Drawing for the job (mm, zero at the part's lowest x, y, z). A direction names the side the tool comes from. Round coordinates to 2 decimals unless told otherwise and drop trailing zeros. Loops run counter-clockwise (first coordinate to the right, second up) from the corner with the lowest first, then second, coordinate; pieces in that order, holes last. Notation, with made-up numbers: M 78,27 L 113,27 A19 cw 113,63 Z; hole C 83.5,7 d3. An arc over 180 degrees is marked long. Use a Markdown table: item, result. Add a question column.
Q1. Pin check, flat tips, straight feed: pin 1 (4 mm diameter, centred on x = 4.5, z = 4, fed in from +Y); pin 2 (0.5 mm diameter, centred on y = 7, z = 3.5, fed in from -X); pin 3 (2.5 mm diameter, centred on x = 2.5, z = 4.5, fed in from +Y). Stop position of each tip, or through.
Q2. Probe line 1 (Y direction, x = 0.75, z = 2); line 2 (X direction, y = 2.25, z = 2.25); line 3 (Y direction, x = 1.5, z = 1.25). List the from-to ranges inside material, lowest first. Write a range as from..to.
Q3. Tool access for the marked faces 4 and 5: list every direction of +Z, -Z, +X, -X, +Y, -Y with a clear straight run to the whole face (end or side of a thin tool).
Q4. Cut at A-A (x = 4.77). Give the cut face in (y, z), plus the area to 3 significant figures.
Q5. Cut at C-C (x = 1.25). Give the cut face in (y, z), plus the area to 3 significant figures.
Q6. Cut at B-B (z = 2.23). Give the cut face in (x, y), plus the area to 3 significant figures.
Q7. Cut at D-D (x = 0.5). Give the cut face in (y, z), plus the area to 3 significant figures.
Q8. Mould opens along X. For the marked faces 1, 2 and 3 say: +X half, -X half, draft (parallel to the pull), parting line (faces both ways), or undercut.
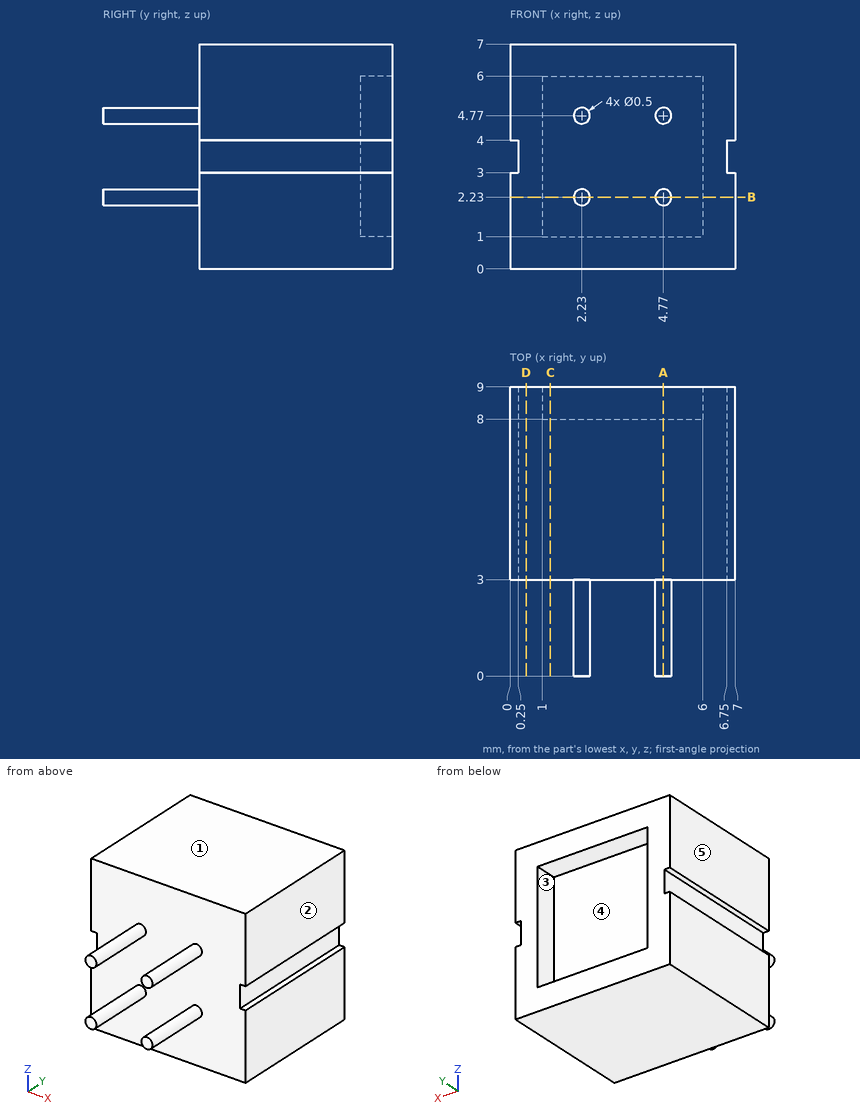
Checked values:
| question | item | result |
|---|---|---|
| 1 | pin 1 | stops at y = 9 |
| 1 | pin 2 | stops at x = 0.25 |
| 1 | pin 3 | stops at y = 8 |
| 2 | line 1 | y = 3..9 |
| 2 | line 2 | x = 1.98..2.48, 4.52..5.02 |
| 2 | line 3 | y = 3..8 |
| 3 | face 4 | +Y |
| 3 | face 5 | +Z, -Z, -X, +Y, -Y |
| 4 | outline | M 0,1.98 L 3,1.98 L 3,0 L 9,0 L 9,1 L 8,1 L 8,6 L 9,6 L 9,7 L 3,7 L 3,5.02 L 0,5.02 L 0,4.52 L 3,4.52 L 3,2.48 L 0,2.48 Z |
| 4 | area | 40.0 mm^2 |
| 5 | outline | M 3,0 L 9,0 L 9,1 L 8,1 L 8,6 L 9,6 L 9,7 L 3,7 Z |
| 5 | area | 37.0 mm^2 |
| 6 | outline | M 0,3 L 1.98,3 L 1.98,0 L 2.48,0 L 2.48,3 L 4.52,3 L 4.52,0 L 5.02,0 L 5.02,3 L 7,3 L 7,9 L 6,9 L 6,8 L 1,8 L 1,9 L 0,9 Z |
| 6 | area | 40.0 mm^2 |
| 7 | outline | M 3,0 L 9,0 L 9,7 L 3,7 Z |
| 7 | area | 42.0 mm^2 |
| 8 | face 1 | draft |
| 8 | face 2 | +X half |
| 8 | face 3 | undercut |
